from build123d import *

# Parameters (mm, degrees)
F1_W     = 70
F1_H     = 25
F1_R     = 5
F2_DEPTH = 10
F3_R     = 6.35


with BuildPart() as f2:
    # F1 (on offset) → F2 (new body)
    with BuildSketch(Plane.XY.offset(25.4)):
        Rectangle(F1_W, F1_H)
        with Locations((-26, 0)):
            Circle(F1_R, mode=Mode.SUBTRACT)
        with Locations((26, 0)):
            Circle(F1_R, mode=Mode.SUBTRACT)
    extrude(amount=F2_DEPTH)

    # F3
    f3_edges = [f2.edges().sort_by_distance(p)[0] for p in [
        (-35, 12.5, 30.4),
        (35, 12.5, 30.4),
        (35, -12.5, 30.4),
        (-35, -12.5, 30.4),
    ]]
    fillet(f3_edges, radius=F3_R)


solid = f2.part
Input: part model. Units: mm. Frame: model coordinates. Round coordinates to 2 decimals unless told otherwise and drop trailing zeros. Loops run counter-clockwise (first coordinate to the right, second up) from the corner with the lowest first, then second, coordinate; pieces in that order, holes last. Notation, with made-up numbers: (13.25, 50) -> (21.25, 50) arc R23 ccw to (21.25, 59) -> close; hole circle Ø6 at (23, 1.25). An arc over 180 degrees is marked (long way). Answer as a JSON object with one key per item and string values. Group by question number.
1) Section query A-A on y = 0. Output: boundary loops of the cut face in (x, z).
2) Ray query, L1, parallel to X at y = -3.25, z = 33.75; L2, parallel to X at y = 0.75, z = 26; L3, parallel to Y at x = -26, z = 29.5. Return the intervals inside material, ascending.
3) Section query C-C on x = 26. Output: boundary loops of the cut face in (y, z), plus the area to 3 significant figures.
4) Pin query (flat end, axial travel): pin 1 (1 mm diameter, centred on y = 8.5, z = 32.5, fed in from +X). Return the tip coordinate at first contact, or that it passes through.
5) Draft query along X for faces 1 (the flat face through (0, 0, 25.4)), 2 (the cylindrical face through (-31, 0, 30)), 3 (the flat face through (35, 0, 30)). Return one class per face: +X half, -X half, draft (parallel to the pull), parting line (faces both ways), or undercut.
6) Section query B-B on z = 34.75. Output: boundary loops of the cut face in (x, y), plus the area to 3 significant figures.
Reply:
{
 "1": {"outline": "(-35, 25.4) -> (-31, 25.4) -> (-31, 35.4) -> (-35, 35.4) -> close; (-21, 25.4) -> (21, 25.4) -> (21, 35.4) -> (-21, 35.4) -> close; (31, 25.4) -> (35, 25.4) -> (35, 35.4) -> (31, 35.4) -> close"},
 "2": {"L1": "x = -35 to -29.8, -22.2 to 22.2, 29.8 to 35", "L2": "x = -35 to -30.94, -21.06 to 21.06, 30.94 to 35", "L3": "y = -12.5 to -5, 5 to 12.5"},
 "3": {"outline": "(-12.5, 25.4) -> (-5, 25.4) -> (-5, 35.4) -> (-12.5, 35.4) -> close; (5, 25.4) -> (12.5, 25.4) -> (12.5, 35.4) -> (5, 35.4) -> close", "area": "150 mm2"},
 "4": {"pin 1": "stops at x = 34.72"},
 "5": {"face 1": "draft", "face 2": "undercut", "face 3": "+X half"},
 "6": {"outline": "(-35, -6.15) arc R6.35 ccw to (-28.65, -12.5) -> (28.65, -12.5) arc R6.35 ccw to (35, -6.15) -> (35, 6.15) arc R6.35 ccw to (28.65, 12.5) -> (-28.65, 12.5) arc R6.35 ccw to (-35, 6.15) -> close; hole circle Ø10 at (-26, 0); hole circle Ø10 at (26, 0)", "area": "1,560 mm2"}
}
